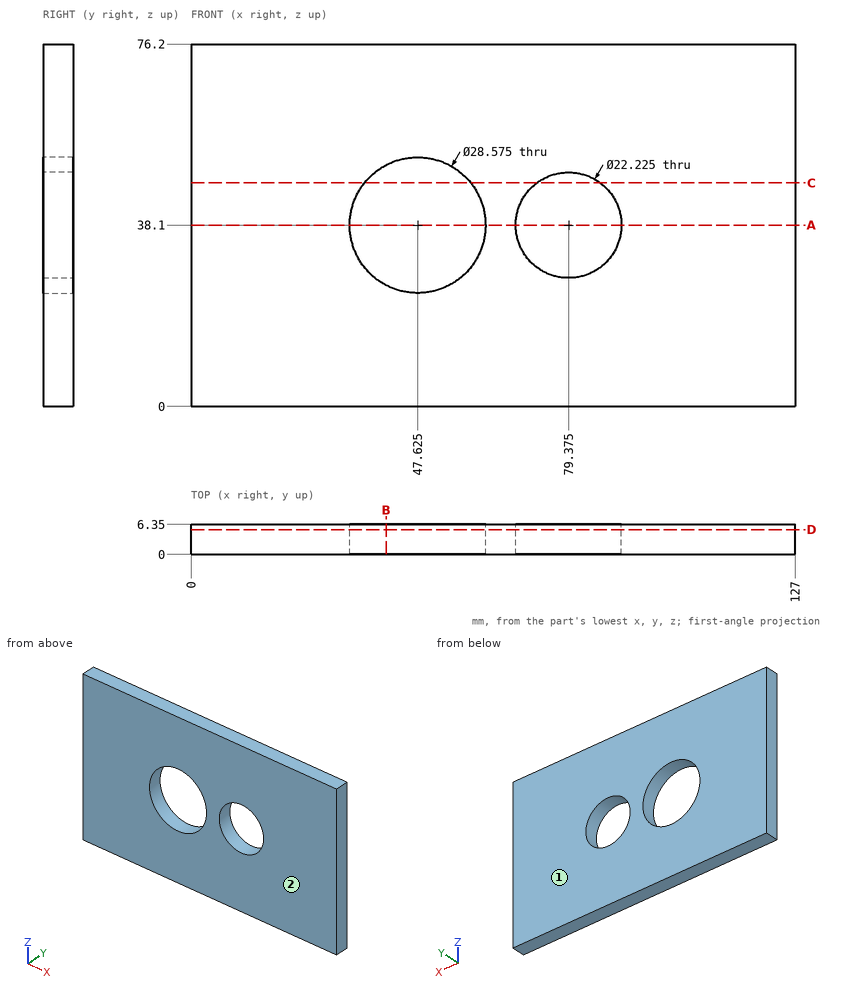
Geometry: see drawing. Coordinates: mm, zero at the bounding-box minimum. Give positions to 0.01 mm unless a question says otherwise; leave off trailing zeros. Order: outer loops, then holes, each group sorted by start corner. A loop starts at its lowest first (then second) coordinate and runs counter-clockwise, first axis right, second up. Notation, with made-up numbers: (-36, 58.5) -> (-25, 58.5) arc R25 ccw to (-25, 83.5) -> close; hole circle Ø11 at (21, 3). An arc over 180 degrees is marked (long way). Write item = value, one per line.
Q1. Cut plane A-A, the plane z = 38.1. Output: boundary loops of the cut face in (x, y), and give its area (3 significant figures).
Data:
outline = (0, 0) -> (33.34, 0) -> (33.34, 6.35) -> (0, 6.35) -> close; (61.91, 0) -> (68.26, 0) -> (68.26, 6.35) -> (61.91, 6.35) -> close; (90.49, 0) -> (127, 0) -> (127, 6.35) -> (90.49, 6.35) -> close
area = 484 mm^2
Q2. Cut plane B-B, the plane x = 41. Output: boundary loops of the cut face in (y, z), and give its area (3 significant figures).
Data:
outline = (0, 0) -> (6.35, 0) -> (6.35, 25.44) -> (0, 25.44) -> close; (0, 50.76) -> (6.35, 50.76) -> (6.35, 76.2) -> (0, 76.2) -> close
area = 323 mm^2
Q3. Material intervals for line 1 (X direction, y = 4, z = 38.1); line 2 (Z direction, x = 58.5, y = 4.25); line 3 (X direction, y = 5, z = 42.5), sorted ascending. Write a range as from..to.
Data:
line_1 = 0..33.34, 61.91..68.26, 90.49..127
line_2 = 0..28.83, 47.37..76.2
line_3 = 0..34.03, 61.22..69.17, 89.58..127
Q4. Cut plane C-C, the plane z = 47. Output: boundary loops of the cut face in (x, y), and give its area (3 significant figures).
Data:
outline = (0, 0) -> (36.45, 0) -> (36.45, 6.35) -> (0, 6.35) -> close; (58.8, 0) -> (72.72, 0) -> (72.72, 6.35) -> (58.8, 6.35) -> close; (86.03, 0) -> (127, 0) -> (127, 6.35) -> (86.03, 6.35) -> close
area = 580 mm^2
Q5. Pull-direction query (Y, two-part tool) for the marked faces 1 and 2; classes: released by +Y, released by -Y, zero draft, split by the parting line, or undercut.
Data:
face_1 = released by +Y
face_2 = released by -Y
Q6. Cut plane D-D, the plane y = 5.25. Output: boundary loops of the cut face in (x, z) (1 decimal).
Data:
outline = (0, 0) -> (127, 0) -> (127, 76.2) -> (0, 76.2) -> close; hole circle Ø28.6 at (47.6, 38.1); hole circle Ø22.2 at (79.4, 38.1)
